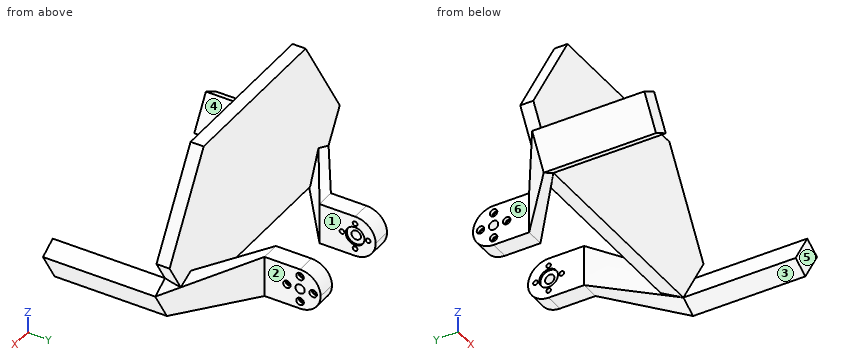
```python
from build123d import *

# Parameters (mm, degrees)
BOSS_EXTRUDE1_DEPTH     = 60
BOSS_EXTRUDE1_2_DEPTH   = 60
BOSS_EXTRUDE2_START     = 30
SKETCH5_W               = 10
SKETCH5_H               = 22
BOSS_EXTRUDE2_DEPTH     = 30
FILLET1_R               = 11
FILLET2_R               = 11
BOSS_EXTRUDE5_DEPTH     = 7
SKETCH12_R              = 5
SKETCH12_R_2            = 2.5
CUT_EXTRUDE1_DEPTH      = 1
SKETCH12_3_R            = 2.5
CUT_EXTRUDE2_DEPTH      = 3
CUT_EXTRUDE8_DEPTH      = 165.032898367
CUT_EXTRUDE8_DEPTH_BACK = 165.032898367
SKETCH16_R              = 2.5
SKETCH17_R              = 1.25
CUT_EXTRUDE9_DEPTH      = 171.03972178
SKETCH17_3_R            = 2
SKETCH17_3_R_2          = 1.25
CUT_EXTRUDE10_DEPTH     = 2


with BuildPart() as part:
    # Sketch4 → Boss-Extrude1 (new body)
    with BuildSketch(Plane(origin=(0, 0, 0), x_dir=(1, 0, 0), z_dir=(0, 1, 0))):
        Polygon((67.506640691, -56.405895144), (76.090203327, -51.275353996), (65.82912103, -34.108228724), (57.245558394, -39.238769873), align=None)
    extrude(amount=-BOSS_EXTRUDE1_DEPTH)



with BuildPart() as body_2:
    # Sketch4 → Boss-Extrude1 2 (new body)
    with BuildSketch(Plane(origin=(0, 0, 0), x_dir=(1, 0, 0), z_dir=(0, 1, 0))):
        Polygon((-57.245558394, -39.238769873), (-67.506640691, -56.405895144), (-76.090203327, -51.275353996), (-65.82912103, -34.108228724), align=None)
    extrude(amount=-BOSS_EXTRUDE1_2_DEPTH)



with BuildPart() as body_3:
    # Sketch5 → Boss-Extrude2 (new body)
    with BuildSketch(Plane(origin=(0, 0, 0), x_dir=(1, 0, 0), z_dir=(0, 1, 0)).offset(BOSS_EXTRUDE2_START)):
        with Locations((-24.245558394, -45.108228724)):
            Rectangle(SKETCH5_W, SKETCH5_H)
    extrude(amount=BOSS_EXTRUDE2_DEPTH)


with BuildPart() as body_2_1:
    add(body_2.part)

    add(body_3.part)  # loft1 joins it to this body
    # loft from a face of the part (loft1)
    loft([body_2_1.faces().sort_by_distance((-66.667880861, 0, 45.257061934))[0], body_2_1.faces().sort_by_distance((-24.245558394, 30, 45.108228724))[0]])


with BuildPart() as body_3_2:
    # Mirror1: mirrored copy
    add(body_2_1.part.mirror(Plane(origin=(0, 0, 0), x_dir=(0, 0, 1), z_dir=(1, 0, 0))))

    # Fillet2
    fillet2_edges = [body_3_2.edges().sort_by_distance(p)[0] for p in [
        (24.245558394, 60, 34.108228724),
        (24.245558394, 60, 56.108228724),
    ]]
    fillet(fillet2_edges, radius=FILLET2_R - 0.0001)  # a hair under: the kernel refuses the full size


with BuildPart() as body_2_2:
    add(body_2_1.part)

    # Fillet1
    fillet1_edges = [body_2_2.edges().sort_by_distance(p)[0] for p in [
        (-24.245558394, 60, 34.108228724),
        (-24.245558394, 60, 56.108228724),
    ]]
    fillet(fillet1_edges, radius=FILLET1_R - 0.0001)  # a hair under: the kernel refuses the full size


with BuildPart() as part_1:
    add(part.part)

    add(body_2_2.part)  # Boss-Extrude5 merges body 2

    add(body_3_2.part)  # Boss-Extrude5 merges body 3 2
    # Sketch11 → Boss-Extrude5 (add)
    with BuildSketch(Plane(origin=(0, 0, 0), x_dir=(1, 0, 0), z_dir=(0, 1, 0))):
        Polygon((75, -68.942529607), (44.93708309, -119.238769873), (-44.93708309, -119.238769873), (-75, -68.942529607), (-57.245558394, -39.238769873), (57.245558394, -39.238769873), align=None)
    extrude(amount=BOSS_EXTRUDE5_DEPTH)

    # Sketch12 → Cut-Extrude1 (cut)
    with BuildSketch(Plane.ZY.offset(-19.245558394)):
        with Locations((45.108228724, 49)):
            Circle(SKETCH12_R)
        with Locations((45.108228724, 49)):
            Circle(SKETCH12_R_2, mode=Mode.SUBTRACT)
    cut_extrude1 = extrude(amount=-CUT_EXTRUDE1_DEPTH, mode=Mode.SUBTRACT)

    # Sketch12<3> → Cut-Extrude2 (cut)
    with BuildSketch(Plane.ZY.offset(-19.245558394)):
        with Locations((45.108228724, 49)):
            Circle(SKETCH12_3_R)
    cut_extrude2 = extrude(amount=-CUT_EXTRUDE2_DEPTH, mode=Mode.SUBTRACT)

    # Sketch16 → Cut-Extrude8 (cut, two sides: drawn at the far end of the back side and taken through both)
    with BuildSketch(Plane.ZY.offset(-19.245558394).offset(-CUT_EXTRUDE8_DEPTH_BACK)):
        with Locations((45.108228724, 49)):
            Circle(SKETCH16_R)
    extrude(amount=CUT_EXTRUDE8_DEPTH + CUT_EXTRUDE8_DEPTH_BACK, mode=Mode.SUBTRACT)

    # Sketch17 → Cut-Extrude9 (cut, through all)
    with BuildSketch(Plane(origin=(29.245558394, 0, 0), x_dir=(0, 0, -1), z_dir=(1, 0, 0))):
        with Locations((-38.108228724, 49)):
            Circle(SKETCH17_R)
        with BuildLine():
            ThreePointArc((-45.108228724, 57.25), (-46.358228724, 56), (-45.108228724, 54.75))
            Line((-45.108228724, 54.75), (-45.108228724, 57.25))
        make_face()
        with BuildLine():
            Line((-45.108228724, 57.25), (-45.108228724, 54.75))
            ThreePointArc((-45.108228724, 54.75), (-44.224345248, 55.116116524), (-43.858228724, 56))
            ThreePointArc((-43.858228724, 56), (-44.224345248, 56.883883476), (-45.108228724, 57.25))
        make_face()
        with Locations((-52.108228724, 49)):
            Circle(SKETCH17_R)
        with Locations((-45.108228724, 42)):
            Circle(SKETCH17_R)
    extrude(amount=-CUT_EXTRUDE9_DEPTH, mode=Mode.SUBTRACT)

    # Sketch17<3> → Cut-Extrude10 (cut)
    # profile 1 of 4: a face of its own
    with BuildSketch(Plane(origin=(29.245558394, 0, 0), x_dir=(0, 0, -1), z_dir=(1, 0, 0))):
        with Locations((-45.108228724, 56)):
            Circle(SKETCH17_3_R)
        with Locations((-45.108228724, 56)):
            Circle(SKETCH17_3_R_2, mode=Mode.SUBTRACT)
    # profile 2 of 4: a face of its own
    with BuildSketch(Plane(origin=(29.245558394, 0, 0), x_dir=(0, 0, -1), z_dir=(1, 0, 0))):
        with Locations((-38.108228724, 49)):
            Circle(SKETCH17_3_R)
        with Locations((-38.108228724, 49)):
            Circle(SKETCH17_3_R_2, mode=Mode.SUBTRACT)
    # profile 3 of 4: a face of its own
    with BuildSketch(Plane(origin=(29.245558394, 0, 0), x_dir=(0, 0, -1), z_dir=(1, 0, 0))):
        with Locations((-45.108228724, 42)):
            Circle(SKETCH17_3_R)
        with Locations((-45.108228724, 42)):
            Circle(SKETCH17_3_R_2, mode=Mode.SUBTRACT)
    # profile 4 of 4: a face of its own
    with BuildSketch(Plane(origin=(29.245558394, 0, 0), x_dir=(0, 0, -1), z_dir=(1, 0, 0))):
        with Locations((-52.108228724, 49)):
            Circle(SKETCH17_3_R)
        with Locations((-52.108228724, 49)):
            Circle(SKETCH17_3_R_2, mode=Mode.SUBTRACT)
    cut_extrude10 = extrude(amount=-CUT_EXTRUDE10_DEPTH, mode=Mode.SUBTRACT)

    # Mirror3: Cut-Extrude1, Cut-Extrude2, Cut-Extrude10 across plane
    add(cut_extrude1.mirror(Plane.ZY), mode=Mode.SUBTRACT)
    add(cut_extrude2.mirror(Plane.ZY), mode=Mode.SUBTRACT)
    add(cut_extrude10.mirror(Plane.ZY), mode=Mode.SUBTRACT)


solid = part_1.part
```
Check sheet for the modelled part. Datum: model origin and axes. Units: mm. Face numbers are marked on the shaded views. A direction names the side the tool comes from. Coordinates: 2 decimals unless noted, no trailing zeros. Order: outer loops, then holes, each group sorted by start corner. A loop starts at its lowest first (then second) coordinate and runs counter-clockwise, first axis right, second up. Notation, with made-up numbers: (17, 35.5) -> (25, 35.5) arc R22 ccw to (25, 43.5) -> close; hole circle Ø4 at (44, -37). An arc over 180 degrees is marked (long way). Write item = value, one per line. Start each with the question number.
1) Material ranges on L1, parallel to Y at x = 27, z = 53; L2, parallel to Y at x = -38.5, z = 116; L3, parallel to X at y = 40, z = 51.5, recorded low to high.
2) Access from +Z, -Z, +X, -X, +Y, -Y to the whole of each face (thin tool, end or side, straight path). Record for the marked faces 1, 2 and 3.
3) Cross-section at D-D (z = 112). Enter the section's corners in (x, y).
4) Mould release check, pull along X, two halves, no side actions. Record for the marked faces 4, 5 and 6: +X half, -X half, draft (parallel to the pull), parting line (faces both ways), or undercut.
5) Cross-section at C-C (z = 90). Enter the section's corners in (x, y), then the cut area to 3 significant figures.
6) Cross-section at B-B (x = -23). State how many separate pieces and enclosed holes the cut face has, then the cut area to 3 significant figures.
7) Cross-section at A-A (y = -10). Enter the section's corners in (x, z).
8) Go/stop test with flat-tipped pins: P1, Ø3, axis at x = -22.5, y = 39, coming from the +Z side; P2, Ø3, axis at y = 50, z = 39, coming from the -X side; P3, Ø5, axis at y = 51, z = 45.5, coming from the +X side. Record where each tip stops, or that it passes through.
Ans:
q1.L1 = 0 to 7, 25.02 to 48.12, 49.88 to 56.66
q1.L2 = 0 to 7
q1.L3 = -29.25 to -19.25, 19.25 to 29.25
q2.face_1 = +Z, -Z, +Y
q2.face_2 = +Z, -Z, +X, +Y
q2.face_3 = -Z, -Y
q3.outline = (-49.26, 0) -> (49.26, 0) -> (49.26, 7) -> (-49.26, 7) -> close
q4.face_4 = undercut
q4.face_5 = draft
q4.face_6 = -X half
q5.outline = (-62.41, 0) -> (62.41, 0) -> (62.41, 7) -> (-62.41, 7) -> close
q5.area = 874 mm²
q6.separate_pieces = 2
q6.enclosed_holes = 5
q6.area = 1,190 mm²
q7.outline = (-76.09, 51.28) -> (-65.83, 34.11) -> (-57.25, 39.24) -> (-67.51, 56.41) -> close; (57.25, 39.24) -> (65.83, 34.11) -> (76.09, 51.28) -> (67.51, 56.41) -> close
q8.P1 = 56.11
q8.P2 = -29.25
q8.P3 = 29.25
